The listing builds one solid part. Answer for the finished solid, in the listing's coordinates (mm). A direction names the side the tool comes from. Give positions to 0.01 mm unless a question says otherwise; leave off trailing zeros. Write each loop counter-clockwise with the first axis right and the second up, starting at its lowest first coordinate (ties: lowest second). Pieces come first, ordered by that corner, then holes. Notation, with made-up numbers: (61.5, 26) -> (65.5, 26) arc R29 ccw to (65.5, 54) -> close; hole circle Ø10 at (2, -19.5). An arc over 180 degrees is marked (long way). Put each result on its own line as item: value. Start each with the question number.
1) For a pull along Z with two mould halves and no side action, classify faces 1 (the flat face through (-7.4, 6, 13.5)), 2 (the flat face through (-8, 6, 16)), 3 (the flat face through (0, 8, 5)) as released by +Z, released by -Z, zero draft, split by the parting line, or undercut.
2) A cutting plane is placed at D-D (z = 8.25). Write down the section's boundary in (x, y).
3) Find the intervals of material crossed by line 1 along X through (y, z) = (9.25, 1.5); line 2 along Z through (x, y) = (-14.5, 17.25); line 3 along Y through (x, z) = (-11.25, 7.5), in increasing order. Write a range as from..to.
4) Flat-ended cylindrical pins translate along their axes: pin 1 Ø8 at (x, y) = (-4, 13.5) entering from +Z; pin 2 Ø1.5 at (x, z) = (-4, 7.5) entering from +Y; pin 3 Ø1 at (x, z) = (-5.5, 13) entering from -Y. Find the tip coordinate at first contact, or state that the pin passes through.
5) A cutting plane is placed at C-C (y = 11.25). Write down the section's boundary in (x, z), then the cut area to 3 significant figures.
6) A cutting plane is placed at A-A (x = -11.75). Write down the section's boundary in (y, z), then the cut area to 3 significant figures.
7) For faces 4 (the flat face through (-10.25, 10, 1)), 5 (the flat face through (-8, 4, 8)), 6 (the flat face through (-7.6, 2, 13.5)), determine the directions among +Z, -Z, +X, -X, +Y, -Y from which every point of the face is accessible in a straight line to the end or side of a thin tool.
8) A cutting plane is placed at B-B (z = 1.5). Write down the section's boundary in (x, y), then the cut area to 3 significant figures.
from build123d import *

# Parameters (mm, degrees)
F0_W      = 15
F0_H      = 20
F1_DEPTH  = 6
F3_DEPTH  = 3
F4_W      = 15
F4_H      = 4
F5_DEPTH  = 5
F5_FACE_W = 15
F5_FACE_H = 4
F7_W      = 15
F7_H      = 4


with BuildPart() as f1:
    # F0 (on Top) → F1 (new body)
    with BuildSketch(Plane.XY):
        with Locations((-7.5, 10)):
            Rectangle(F0_W, F0_H)
    extrude(amount=F1_DEPTH)

    # F2 (on face) → F3 (cut)
    with BuildSketch(Plane(origin=(0, 0, 0), x_dir=(1, 0, 0), z_dir=(0, 0, -1))):
        Polygon((-7.5, -15.25), (-4.75, -15.25), (-4.75, -4.75), (-7.5, -4.75), (-10.25, -4.75), (-10.25, -15.25), align=None)
    extrude(amount=-F3_DEPTH, mode=Mode.SUBTRACT)

    # F4 (on face) → F5 (join)
    with BuildSketch(Plane.XY.offset(6)):
        with Locations((-7.5, 2)):
            Rectangle(F4_W, F4_H)
    extrude(amount=F5_DEPTH)

    # F5_face (on face) → F8 section 0
    with BuildSketch(Plane(origin=(-7.5, 2, 11), x_dir=(1, 0, 0), z_dir=(0, 0, 1))):
        Rectangle(F5_FACE_W, F5_FACE_H)
    # F7 (on offset) → F8 section 1
    with BuildSketch(Plane.XY.offset(16)):
        with Locations((-7.5, 6)):
            Rectangle(F7_W, F7_H)
    loft()


solid = f1.part
Reply:
1. face 1: undercut
1. face 2: released by +Z
1. face 3: zero draft
2. outline: (-15, 0) -> (0, 0) -> (0, 4) -> (-15, 4) -> close
3. line 1: x = -15..-10.25, -4.75..0
3. line 2: z = 0..6
3. line 3: y = 0..4
4. pin 1: stops at z = 6
4. pin 2: stops at y = 4
4. pin 3: stops at y = 1.2
5. outline: (-15, 0) -> (-10.25, 0) -> (-10.25, 3) -> (-4.75, 3) -> (-4.75, 0) -> (0, 0) -> (0, 6) -> (-15, 6) -> close
5. area: 73.5 mm2
6. outline: (0, 0) -> (20, 0) -> (20, 6) -> (4, 6) -> (4, 11) -> (8, 16) -> (4, 16) -> (0, 11) -> close
6. area: 160 mm2
7. face 4: -Z
7. face 5: +X, -X, +Y
7. face 6: +Z, +X, -X, -Y
8. outline: (-15, 0) -> (0, 0) -> (0, 20) -> (-15, 20) -> close; hole (-10.25, 4.75) -> (-4.75, 4.75) -> (-4.75, 15.25) -> (-10.25, 15.25) -> close
8. area: 242 mm2
